Part model, mm, in its own coordinate system. A direction names the side the tool comes from. Coordinates: 2 decimals unless noted, no trailing zeros. Loops run counter-clockwise (first coordinate to the right, second up) from the corner with the lowest first, then second, coordinate; pieces in that order, holes last. Notation, with made-up numbers: (-3, 33) - (53, 33) arc R21 cw to (53, 61) - close; hole circle Ø1 at (-2, 50). An arc over 180 degrees is marked (long way). Use a Markdown table: item, result. Add a question column.
1. Band-saw the part on D-D, the plane z = 4. Give the cut face in (x, y) (1 decimal), plus the area to 3 significant figures.
2. Band-saw the part on A-A, the plane z = 5.5. Give the cut face in (x, y) (1 decimal), plus the area to 3 significant figures.
3. Wall check: probe 1 along Y at (x, z) = (-0.75, 4.75) (3 decimals); probe 2 along Y at (x, z) = (1, 11.25); probe 3 along Y at (x, z) = (0.5, 8) (3 decimals). Give the ranges that are in metal, low to high. Write a range as [from, to].
4. Band-saw the part on C-C, the plane y = 4. Give the cut face in (x, z) (1 decimal), plus the area to 3 significant figures.
5. Pull direction Z, two halves, no side cores. Call faces 6 (the flat face through (0, -9.525, 6)), 7 (the cylindrical face through (0.022, -17.691, 0.764)), 8 (the flat face through (-0.022, -9.847, 12.247)): pulls with the +Z half, pulls with the -Z half, needs draft (parallel to the pull), parting line crosses it, or undercut.
6. Drop flat-ended pins along their axis: pin 1 (1.1 mm diameter, centred on x = 0, z = 11.5, fed in from +Y); pin 2 (1 mm diameter, centred on x = -0.5, z = 7.5, fed in from +Y); pin 3 (0.9 mm diameter, centred on x = 0.5, y = 15, fed in from +Z) (3 decimals); pin 4 (1 mm diameter, centred on x = -0.5, y = -1.5, fed in from +Z) (3 decimals). Give the stop position or say it passes through.
7. 3-axis set-ups, long thin cutter, end or side, ignore diameter. For faces 1 (the cylindrical face through (0, -7.2, 3.5)), 2 (the flat face through (0, -15, 9.525)), 3 (the flat face through (0, 9, 12.827)), 4 (the flat face through (0, 15, 9.525)), 5 (the flat face through (0, 9.525, 6)): which of +Z, -Z, +X, -X, +Y, -Y reach the whole face in a straight line?
from build123d import *

# Parameters (mm, degrees)
SKETCH1_W      = 3.175
SKETCH1_H      = 36.83
BASE_DEPTH     = 3.175
SKETCH3_W      = 6.35
SKETCH3_H      = 5.715
RETAINER_DEPTH = 3.175
TAB_DEPTH      = 3.175
FILLET1_R      = 1.27
FILLET2_R      = 2.54
CHAMFER1_SIZE  = 2.032


with BuildPart() as part:
    # Sketch1 → Base (new body)
    with BuildSketch(Plane.XY):
        Rectangle(SKETCH1_W, SKETCH1_H)
    extrude(amount=BASE_DEPTH)

    # Sketch3 → Retainer (add)
    with BuildSketch(Plane.ZY.offset(1.5875)):
        with Locations((6.35, 15.5575)):
            Rectangle(SKETCH3_W, SKETCH3_H)
        with Locations((6.35, -15.5575)):
            Rectangle(SKETCH3_W, SKETCH3_H)
    extrude(amount=-RETAINER_DEPTH)

    # Sketch5 → Tab (add)
    with BuildSketch(Plane.ZY.offset(1.5875)):
        Polygon((3.175, 9.525), (9.525, 9.525), (10.668, 10.16), (11.684, 10.16), (12.827, 9.525), (12.827, 7.62), (3.175, 7.62), align=None)
        Polygon((12.827, -7.62), (3.175, -7.62), (3.175, -9.525), (9.525, -9.525), (10.668, -10.16), (11.684, -10.16), (12.827, -9.525), align=None)
    extrude(amount=-TAB_DEPTH)

    # Fillet1
    fillet1_edges = [part.edges().sort_by_distance(p)[0] for p in [
        (0, 7.62, 3.175),
        (0, -7.62, 3.175),
    ]]
    fillet(fillet1_edges, radius=FILLET1_R)

    # Fillet2
    fillet2_edges = [part.edges().sort_by_distance(p)[0] for p in [
        (0, 18.415, 9.525),
        (0, -18.415, 9.525),
        (0, -18.415, 0),
        (0, 18.415, 0),
    ]]
    fillet(fillet2_edges, radius=FILLET2_R)

    # Chamfer1
    chamfer1_edges = [part.edges().sort_by_distance(p)[0] for p in [
        (0, 12.7, 9.525),
        (0, -12.7, 9.525),
    ]]
    chamfer(chamfer1_edges, length=CHAMFER1_SIZE)


solid = part.part
Geometry check:
| question | item | result |
|---|---|---|
| 1 | outline | (-1.6, -18.4) - (1.6, -18.4) - (1.6, -12.7) - (-1.6, -12.7) - close; (-1.6, -9.5) - (1.6, -9.5) - (1.6, -7.5) - (-1.6, -7.5) - close; (-1.6, 7.5) - (1.6, 7.5) - (1.6, 9.5) - (-1.6, 9.5) - close; (-1.6, 12.7) - (1.6, 12.7) - (1.6, 18.4) - (-1.6, 18.4) - close |
| 1 | area | 48.9 mm^2 |
| 2 | outline | (-1.6, -18.4) - (1.6, -18.4) - (1.6, -12.7) - (-1.6, -12.7) - close; (-1.6, -9.5) - (1.6, -9.5) - (1.6, -7.6) - (-1.6, -7.6) - close; (-1.6, 7.6) - (1.6, 7.6) - (1.6, 9.5) - (-1.6, 9.5) - close; (-1.6, 12.7) - (1.6, 12.7) - (1.6, 18.4) - (-1.6, 18.4) - close |
| 2 | area | 48.4 mm^2 |
| 3 | probe 1 | y = [-18.415, -12.7], [-9.525, -7.62], [7.62, 9.525], [12.7, 18.415] |
| 3 | probe 2 | y = [-10.16, -7.62], [7.62, 10.16] |
| 3 | probe 3 | y = [-18.203, -13.207], [-9.525, -7.62], [7.62, 9.525], [13.207, 18.203] |
| 4 | outline | (-1.6, 0) - (1.6, 0) - (1.6, 3.2) - (-1.6, 3.2) - close |
| 4 | area | 10.1 mm^2 |
| 5 | face 6 | undercut |
| 5 | face 7 | pulls with the -Z half |
| 5 | face 8 | pulls with the +Z half |
| 6 | pin 1 | stops at y = 10.16 |
| 6 | pin 2 | stops at y = 18.41 |
| 6 | pin 3 | stops at z = 9.525 |
| 6 | pin 4 | stops at z = 3.175 |
| 7 | face 1 | +Z, +X, -X |
| 7 | face 2 | +Z, +X, -X, -Y |
| 7 | face 3 | +Z, +X, -X, +Y, -Y |
| 7 | face 4 | +Z, +X, -X, +Y |
| 7 | face 5 | +X, -X |
